```python
from build123d import *

# Parameters (mm, degrees)
SKETCH1_W           = 215.9
SKETCH1_H           = 114.3
BOSS_EXTRUDE1_DEPTH = 30.17
SKETCH2_W           = 15.5
SKETCH2_H           = 110.06
CUT_EXTRUDE1_DEPTH  = 8.5
SKETCH3_R           = 26
BOSS_EXTRUDE2_DEPTH = 1


with BuildPart() as part:
    # Sketch1 → Boss-Extrude1 (new body)
    with BuildSketch(Plane(origin=(0, 0, 0), x_dir=(1, 0, 0), z_dir=(0, 1, 0))):
        with Locations((107.95, 57.15)):
            Rectangle(SKETCH1_W, SKETCH1_H)
    extrude(amount=BOSS_EXTRUDE1_DEPTH)

    # Sketch2 → Cut-Extrude1 (cut)
    with BuildSketch(Plane(origin=(0, 30.17, 0), x_dir=(1, 0, 0), z_dir=(0, 1, 0))):
        with Locations((7.75, 57.15)):
            Rectangle(SKETCH2_W, SKETCH2_H)
    extrude(amount=-CUT_EXTRUDE1_DEPTH, mode=Mode.SUBTRACT)

    # Sketch3 → Boss-Extrude2 (add)
    with BuildSketch(Plane(origin=(0, 30.17, 0), x_dir=(1, 0, 0), z_dir=(0, 1, 0))):
        with Locations((168.4, 78.3)):
            Circle(SKETCH3_R)
    extrude(amount=BOSS_EXTRUDE2_DEPTH)


solid = part.part
```
Part model, mm, in its own coordinate system. A direction names the side the tool comes from. Give positions to 0.01 mm unless a question says otherwise; leave off trailing zeros. Write each loop counter-clockwise with the first axis right and the second up, starting at its lowest first coordinate (ties: lowest second). Pieces come first, ordered by that corner, then holes. Notation, with made-up numbers: (11, -37.75) -> (50, -37.75) arc R19 cw to (50, -2.75) -> close; hole circle Ø2 at (58, 3.5). An arc over 180 degrees is marked (long way). Put each result on its own line as item: value. Start each with the question number.
Item 1: Cut at C-C (x = 190). List the corners of the cut face in (y, z).
Item 2: Cut at A-A (x = 168.4). List the corners of the cut face in (y, z).
Item 3: Wall check: L1, parallel to Z at x = 12, y = 28.5; L2, parallel to Y at x = 136, z = -89.5; L3, parallel to X at y = 29.5, z = -83. Give the ranges that are in metal, low to high. Write a range as [from, to].
Item 4: Which spindle directions (+Z, -Z, +X, -X, +Y, -Y) get a long thin tool onto all of the face, cutting with end or side? Do faces 4 (the face through (106, 15, -114.3)), 5 (the face through (8, 26, -112.18)). Say none if no direction does.
Item 5: Cut at D-D (z = -29). List the corners of the cut face in (x, y), then the cut area to 3 significant figures.
Item 6: Pull direction Z, two halves, no side cores. Call faces 1 (the face through (106, 0, -58)), 2 (the face through (15.5, 26, -56)), 3 (the face through (142.425, 30.663, -79.443)): pulls with the +Z half, pulls with the -Z half, needs draft (parallel to the pull), parting line crosses it, or undercut.
Item 7: Pin check, flat tips, straight feed: pin 1 Ø9.5 at (y, z) = (27, -80.5) entering from -X; pin 2 Ø6 at (x, z) = (114, -47.5) entering from +Y; pin 3 Ø17 at (x, z) = (6.5, -44.5) entering from +Y. Stop position of each tip, or through.
Item 8: Cut at B-B (z = -78.3). List the corners of the cut face in (x, y).
Answer list:
1. outline: (0, -114.3) -> (30.17, -114.3) -> (30.17, -92.77) -> (31.17, -92.77) -> (31.17, -63.83) -> (30.17, -63.83) -> (30.17, 0) -> (0, 0) -> close
2. outline: (0, -114.3) -> (30.17, -114.3) -> (30.17, -104.3) -> (31.17, -104.3) -> (31.17, -52.3) -> (30.17, -52.3) -> (30.17, 0) -> (0, 0) -> close
3. L1: z = [-114.3, -112.18], [-2.12, 0]
3. L2: y = [0, 30.17]
3. L3: x = [15.5, 215.9]
4. face 4: -Z, +X, -X, +Y, -Y
4. face 5: -X, +Y
5. outline: (0, 0) -> (215.9, 0) -> (215.9, 30.17) -> (15.5, 30.17) -> (15.5, 21.67) -> (0, 21.67) -> close
5. area: 6,380 mm2
6. face 1: needs draft
6. face 2: undercut
6. face 3: parting line crosses it
7. pin 1: stops at x = 15.5
7. pin 2: stops at y = 30.17
7. pin 3: stops at y = 21.67
8. outline: (0, 0) -> (215.9, 0) -> (215.9, 30.17) -> (194.4, 30.17) -> (194.4, 31.17) -> (142.4, 31.17) -> (142.4, 30.17) -> (15.5, 30.17) -> (15.5, 21.67) -> (0, 21.67) -> close
